Source: three-view drawing plus pictorial views. Frame: mm from the lowest corner of the part. A direction names the side the tool comes from. Round coordinates to 2 decimals unless told otherwise and drop trailing zeros. Order: outer loops, then holes, each group sorted by start corner. A loop starts at its lowest first (then second) coordinate and runs counter-clockwise, first axis right, second up. Notation, with made-up numbers: M -5,26 L 21,26 A35 cw 21,63 Z; hole C 87.5,-1 d8. An arc over 180 degrees is marked long. Return JSON: item names as keys, results as strings. Group by question number.
Q1. Cut plane C-C on z = 23.5. Output: boundary loops of the cut face in (x, y).
Q2. Cut plane D-D on y = 9. Output: boundary loops of the cut face in (x, z), and give its area (3 significant figures).
Q3. Mould query, pull axis X, two halves, no side actions, for the marked faces 4 and 5. Classes: released by +X, released by -X, zero draft, split by the parting line, or undercut.
Q4. Ray query, probe 1 along X at (y, z) = (7, 18); probe 2 along Y at (x, z) = (14.5, 5.5); probe 3 along X at (y, z) = (12, 22). Return the intervals inside material, ascending.
Q5. Contact query for flat-ended pins moving along their axis: pin 1 (10 mm diameter, centred on x = 11.5, z = 29, fed in from +Y); pin 2 (2 mm diameter, centred on y = 27, z = 17, fed in from -X); pin 3 (5 mm diameter, centred on x = 45.5, y = 8.5, fed in from +Z); pin 4 (8 mm diameter, centred on x = 65, y = 31.5, fed in from -Z). Output: stop coordinate, or through.
Q6. Cut plane B-B on y = 21.5. Output: boundary loops of the cut face in (x, z), and give its area (3 significant figures).
Q7. Access query for the marked faces 1, 2 and 3. Directions: +Z, -Z, +X, -X, +Y, -Y. A direction counts if a zero-diameter tool reaches every point of the face in a straight line with its end or side. Return the directions, or none.
Q8. Cut plane A-A on x = 82.5. Output: boundary loops of the cut face in (y, z), and give its area (3 significant figures).
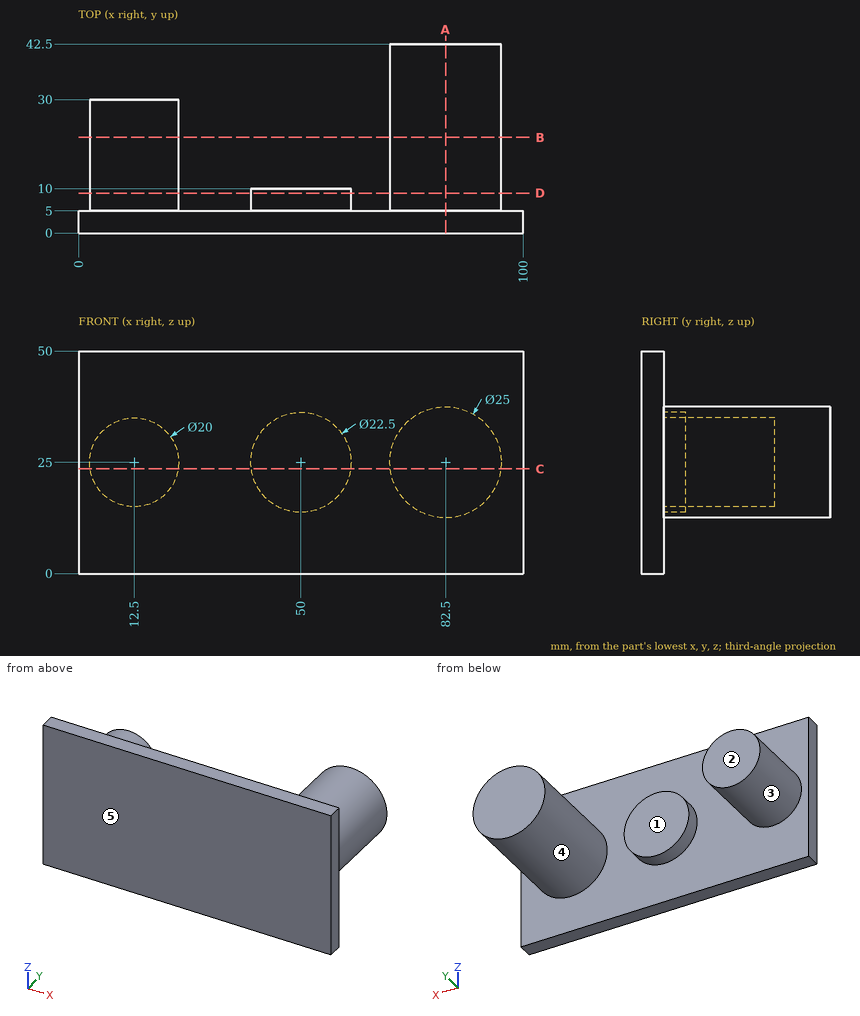
Result sheet:
{
 "1": {"outline": "M 0,0 L 100,0 L 100,5 L 94.91,5 L 94.91,42.5 L 70.09,42.5 L 70.09,5 L 61.15,5 L 61.15,10 L 38.85,10 L 38.85,5 L 22.39,5 L 22.39,30 L 2.61,30 L 2.61,5 L 0,5 Z"},
 "2": {"outline": "C 12.5,25 d20; C 50,25 d22.5; C 82.5,25 d25", "area": "1,200 mm²"},
 "3": {"face 4": "undercut", "face 5": "zero draft"},
 "4": {"probe 1": "x = 5.36 to 19.64, 41.19 to 58.81, 72.14 to 92.86", "probe 2": "y = 0 to 5", "probe 3": "x = 2.96 to 22.04, 70.37 to 94.63"},
 "5": {"pin 1": "stops at y = 30", "pin 2": "stops at x = 5.36", "pin 3": "stops at z = 36.07", "pin 4": "passes through"},
 "6": {"outline": "C 12.5,25 d20; C 82.5,25 d25", "area": "805 mm²"},
 "7": {"face 1": "+Z, -Z, +Y", "face 2": "+Z, -Z, -X, +Y", "face 3": "+Y"},
 "8": {"outline": "M 0,0 L 5,0 L 5,12.5 L 42.5,12.5 L 42.5,37.5 L 5,37.5 L 5,50 L 0,50 Z", "area": "1,190 mm²"}
}
